Input: part model. Units: mm. Frame: model coordinates. A direction names the side the tool comes from. Round coordinates to 2 decimals unless told otherwise and drop trailing zeros. Loops run counter-clockwise (first coordinate to the right, second up) from the corner with the lowest first, then second, coordinate; pieces in that order, holes last. Notation, with made-up numbers: (18.25, 3) - (30.25, 3) arc R17 ccw to (30.25, 23) - close; hole circle Ø9 at (27.25, 23.25). An arc over 180 degrees is marked (long way). Use CSV: the item, a comma, the result in double quotes. Start each with the question number.
1. Access query for faces 1 (the flat face through (0, 10, 29)), 2 (the flat face through (-18, 10, 28)), 3 (the flat face through (46, 3, -33)), 4 (the flat face through (36, 10, -14)), 5 (the flat face through (-43, 3, 28)). Directions: +Z, -Z, +X, -X, +Y, -Y. A direction counts if a zero-diameter tool reaches every point of the face in a straight line with its end or side. Return the directions, or none.
2. Material intervals for probe 1 along X at (y, z) = (3.9, -34); probe 2 along X at (y, z) = (2.9, 34); probe 3 along Z at (x, y) = (-27.5, 10.75), sorted ascending. Write a range as from..to.
3. Cut plane A-A (z = -34). Return loops of the section in (x, y), and give its area (3 significant figures).
4. Cut plane B-B (x = 42). Return loops of the section in (y, z).
5. Cut plane C-C (z = 34). Return loops of the section in (x, y).
6. Pull-direction query (Z, two-part tool) for faces 6 (the cylindrical face through (-43.71, 2.96, 34.38)), 7 (the flat face through (-41, 3, -38)), 8 (the flat face through (-40, 6, 33)), 9 (the flat face through (-36, 10, 0)); classes: +Z half, -Z half, draft (parallel to the pull), parting line (faces both ways), or undercut.
7. Pin query (flat end, axial travel): P1, Ø3, axis at y = 3.5, z = 35, coming from the +X side; P2, Ø3.5, axis at y = 11, z = 30, coming from the +X side; P3, Ø2, axis at x = -42, z = 34, coming from the -Y side; P4, Ø6.5, axis at x = 43, y = 3, coming from the +Z side. Return the tip coordinate at first contact, or that it passes through.
8. Cut plane D-D (x = -42). Return loops of the section in (y, z).
```python
from build123d import *

# Parameters (mm, degrees)
EXTRUDE_1_DEPTH = 20
SKETCH_2_W      = 10
SKETCH_2_H      = 10
SKETCH_2_R      = 1.75
EXTRUDE_2_DEPTH = 6


with BuildPart() as part:
    # 草图1 → 凸台-拉伸1 (new body)
    with BuildSketch(Plane(origin=(0, 0, 0), x_dir=(1, 0, 0), z_dir=(0, 1, 0))):
        Polygon((0, -28), (0, -31), (-39, -31), (-39, 31), (39, 31), (39, 0), (36, 0), (36, 28), (-36, 28), (-36, -28), align=None)
    extrude(amount=EXTRUDE_1_DEPTH)

    # 草图2 → 凸台-拉伸2 (add)
    # profile 1 of 3: a face of its own
    with BuildSketch(Plane.XZ):
        with Locations((-41, 33)):
            Rectangle(SKETCH_2_W, SKETCH_2_H)
        with Locations(Location((-42, 34, 0), (0, 0, 270))):
            Circle(SKETCH_2_R, mode=Mode.SUBTRACT)
    # profile 2 of 3: a face of its own
    with BuildSketch(Plane.XZ):
        with Locations((-41, -33)):
            Rectangle(SKETCH_2_W, SKETCH_2_H)
        with Locations(Location((-42, -34, 0), (0, 0, 90))):
            Circle(SKETCH_2_R, mode=Mode.SUBTRACT)
    # profile 3 of 3: a face of its own
    with BuildSketch(Plane.XZ):
        with Locations((41, -33)):
            Rectangle(SKETCH_2_W, SKETCH_2_H)
        with Locations(Location((42, -34, 0), (0, 0, 270))):
            Circle(SKETCH_2_R, mode=Mode.SUBTRACT)
    extrude(amount=-EXTRUDE_2_DEPTH)


solid = part.part
```
Established:
1,face 1,"+Z, +X, +Y, -Y"
1,face 2,"+X, +Y, -Y"
1,face 3,"+Z, -Z, +X, +Y, -Y"
1,face 4,"+Z, +Y, -Y"
1,face 5,"-X, +Y, -Y"
2,probe 1,"x = -46..-43.75, -40.25..-36, 36..40.25, 43.75..46"
2,probe 2,"x = -46..-43.75, -40.25..-36"
2,probe 3,"z = -31..-28, 28..31"
3,outline,"(-46, 0) - (-43.75, 0) - (-43.75, 6) - (-46, 6) - close; (-40.25, 0) - (-36, 0) - (-36, 6) - (-40.25, 6) - close; (36, 0) - (40.25, 0) - (40.25, 6) - (36, 6) - close; (43.75, 0) - (46, 0) - (46, 6) - (43.75, 6) - close"
3,area,"78.0 mm2"
4,outline,"(0, -38) - (6, -38) - (6, -35.75) - (0, -35.75) - close; (0, -32.25) - (6, -32.25) - (6, -28) - (0, -28) - close"
5,outline,"(-46, 0) - (-43.75, 0) - (-43.75, 6) - (-46, 6) - close; (-40.25, 0) - (-36, 0) - (-36, 6) - (-40.25, 6) - close"
6,face 6,"undercut"
6,face 7,"-Z half"
6,face 8,"draft"
6,face 9,"undercut"
7,P1,"stops at x = -36"
7,P2,"stops at x = 0"
7,P3,"passes through"
7,P4,"stops at z = -28"
8,outline,"(0, -38) - (6, -38) - (6, -35.75) - (0, -35.75) - close; (0, -32.25) - (6, -32.25) - (6, -28) - (0, -28) - close; (0, 28) - (6, 28) - (6, 32.25) - (0, 32.25) - close; (0, 35.75) - (6, 35.75) - (6, 38) - (0, 38) - close"
